Drawing for the job (mm, zero at the part's lowest x, y, z). A direction names the side the tool comes from. Give positions to 0.01 mm unless a question says otherwise; leave off trailing zeros. Order: outer loops, then holes, each group sorted by start corner. A loop starts at its lowest first (then second) coordinate and runs counter-clockwise, first axis right, second up. Notation, with made-up numbers: (33, -12.5) - (71, -12.5) arc R33 ccw to (71, 21.5) - close; hole circle Ø2 at (42, 78). An arc over 180 degrees is marked (long way). Use a Markdown table: item, result.
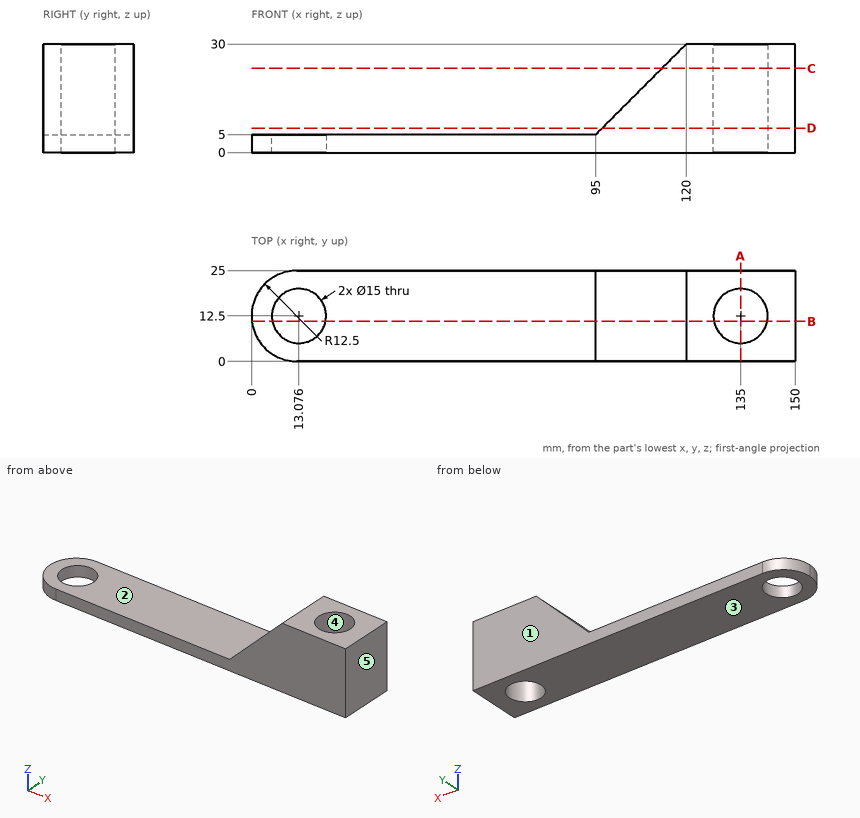
1) Tool access for the marked faces 1 and 2: list every direction of +Z, -Z, +X, -X, +Y, -Y with a clear straight run to the whole face (end or side of a thin tool).
Computed:
| item | result |
|---|---|
| face 1 | +Z, -Z, +X, -X, +Y |
| face 2 | +Z, -X, +Y, -Y |
2) Wall check: line 1 (Y direction, x = 135, z = 15); line 2 (Z direction, x = 32, y = 4.5); line 3 (X direction, y = 15.5, z = 7.5) (1 decimal). Give the ranges that are in metal, low to high. Write a range as from..to.
Computed:
| item | result |
|---|---|
| line 1 | y = 0..5, 20..25 |
| line 2 | z = 0..5 |
| line 3 | x = 97.5..128.1, 141.9..150 |
3) Slice it at B-B (y = 11). Write the cut outline in (x, z), and give its area (3 significant figures).
Computed:
| item | result |
|---|---|
| outline | (0.09, 0) - (5.73, 0) - (5.73, 5) - (0.09, 5) - close; (20.42, 0) - (127.65, 0) - (127.65, 30) - (120, 30) - (95, 5) - (20.42, 5) - close; (142.35, 0) - (150, 0) - (150, 30) - (142.35, 30) - close |
| area | 1,300 mm² |
4) Pin check, flat tips, straight feed: P1, Ø12.5, axis at x = 27.5, y = 14, coming from the +Z side; P2, Ø5, axis at y = 6, z = 3, coming from the -X side; P3, Ø12, axis at y = 9, z = 13, coming from the -X side. Stop position of each tip, or through.
Computed:
| item | result |
|---|---|
| P1 | stops at z = 5 |
| P2 | stops at x = 0.66 |
| P3 | stops at x = 97 |
5) Slice it at D-D (z = 6.75). Write the cut outline in (x, y).
Computed:
| item | result |
|---|---|
| outline | (96.75, 0) - (150, 0) - (150, 25) - (96.75, 25) - close; hole circle Ø15 at (135, 12.5) |
6) Slice it at C-C (z = 23.25). Write the cut outline in (x, y).
Computed:
| item | result |
|---|---|
| outline | (113.25, 0) - (150, 0) - (150, 25) - (113.25, 25) - close; hole circle Ø15 at (135, 12.5) |
7) Two-plate mould, pull along X, no slides. Class the marked faces 3, 4 and 5: +X half, -X half, draft (parallel to the pull), parting line (faces both ways), or undercut.
Computed:
| item | result |
|---|---|
| face 3 | draft |
| face 4 | undercut |
| face 5 | +X half |
8) Slice it at A-A (x = 135). Write the cut outline in (y, z).
Computed:
| item | result |
|---|---|
| outline | (0, 0) - (5, 0) - (5, 30) - (0, 30) - close; (20, 0) - (25, 0) - (25, 30) - (20, 30) - close |
